Geometry: final body of the model. Coordinates: model frame, mm. A direction names the side the tool comes from. Round coordinates to 2 decimals unless told otherwise and drop trailing zeros. Order: outer loops, then holes, each group sorted by start corner. A loop starts at its lowest first (then second) coordinate and runs counter-clockwise, first axis right, second up. Notation, with made-up numbers: (34.25, -10.75) -> (61.25, -10.75) arc R23 ccw to (61.25, 9.25) -> close; hole circle Ø6 at (41.25, 7.25). An arc over 180 degrees is marked (long way). Put each result on its own line as item: value.
```python
from build123d import *

# Parameters (mm, degrees)
SHELL5_T         = 1
SWEEP1_PROFILE_R = 2.5


with BuildPart() as part:
    # Sketch1 → Revolve1 (revolve)
    with BuildSketch(Plane.XY, mode=Mode.PRIVATE) as revolve1_sk:
        Polygon((0, 620), (-126, 620), (-126, 610.763571771), (-131.422468228, 610.763571771), (-131.422468228, 606.763571771), (-126.257555316, 606.763571771), (-126.257555316, 591.763571771), (-131.422468228, 591.763571771), (-131.422468228, 587.763571771), (-126.257555316, 587.763571771), (-111.609923626, 0), (0, 0), align=None)
    revolve(revolve1_sk.sketch.rotate(Axis((0, 0, 0), (0, 1, 0)), 270), axis=Axis((0, 0, 0), (0, 1, 0)))

    # Shell5
    shell5_openings = [part.faces().sort_by_distance(p)[0] for p in [
        (0, 620, 0),
    ]]
    offset(amount=SHELL5_T, openings=shell5_openings, kind=Kind.INTERSECTION)

    # Sweep1: sweep along a path in Sketch4
    with BuildLine(Plane(origin=(0, 0, 0), x_dir=(1, 0, 0), z_dir=(0, 0, -1))) as sweep1_path:
        Line((-14.999820713, 0), (-14.999820713, -280.07351805))
        ThreePointArc((-14.999820713, -280.07351805), (0, -295.073338764), (14.999820713, -280.07351805))
        Line((14.999820713, -280.07351805), (14.999820713, -0.073338764))
    # Sweep1 profile (on start of the path) → Sweep1 (sweep)
    with BuildSketch(Plane(origin=(-14.999820713, 0, 0), x_dir=(1, 0, 0), z_dir=(0, 1, 0))):
        Circle(SWEEP1_PROFILE_R)
    sweep(path=sweep1_path.line)


solid = part.part
```
1. Cut plane B-B on y = 370.5. Return loops of the section in (x, z), and give its area (3 significant figures).
Ans:
outline: circle Ø243.69 at (0, 0); hole circle Ø241.69 at (0, 0)
area: 763 mm²
2. Cut plane C-C on y = 103. Return loops of the section in (x, z), and give its area (3 significant figures).
Ans:
outline: circle Ø230.35 at (0, 0); circle Ø5 at (-15, 0); circle Ø5 at (15, 0); hole circle Ø228.35 at (0, 0)
area: 760 mm²
3. Cut plane A-A on y = 263. Return loops of the section in (x, z), and give its area (3 significant figures).
Ans:
outline: circle Ø238.33 at (0, 0); circle Ø5 at (-15, 0); circle Ø5 at (15, 0); hole circle Ø236.33 at (0, 0)
area: 785 mm²
4. Contact query for flat-ended pins moving along their axis: P1, Ø2, axis at x = -25.5, y = 489.5, coming from the +Z side; P2, Ø2, axis at y = 170, z = -30.5, coming from the +X side; P3, Ø2, axis at y = 133.5, z = -28.5, coming from the -X side. Output: stop coordinate, or through.
Ans:
P1: z = 122.38
P2: x = 113.06
P3: x = -112.63
5. Draft query along Z for faces 5 (the face through (-126.175, 599.173, 16.566)), 6 (the face through (-2, -1, 2)), 7 (the face through (-117, 591.764, -49)). Return one class per face: +Z half, -Z half, draft (parallel to the pull), parting line (faces both ways), or undercut.
Ans:
face 5: parting line
face 6: draft
face 7: undercut
6. Set-up query: faces 1 (the face through (-131.3, 589.7, 17.2)), 2 (the face through (127, 611.764, 9)), 3 (the face through (116.96, 288.77, 25.97)), 4 (the face through (-69, 592.764, -109)). Return all of +Z, -Z, +X, -X, +Y, -Y with unobstructed straight access to the full face (end or side cutting, diameter ignored); none if empty.
Ans:
face 1: +Y, -Y
face 2: +Y
face 3: -Y
face 4: none
7. Material intervals for probe 1 along X at (y, z) = (614.75, 0); probe 2 along X at (y, z) = (608, 0); probe 3 along X at (y, z) = (97.5, -1), sorted ascending.
Ans:
probe 1: -127 to -126, 126 to 127
probe 2: -132.42 to -131.42, 131.42 to 132.42
probe 3: -115.04 to -114.04, -17.29 to -12.71, 12.71 to 17.29, 114.04 to 115.04
8. Cut plane D-D on y = 535.5. Return loops of the section in (x, z), and give its area (3 significant figures).
Ans:
outline: circle Ø251.91 at (0, 0); hole circle Ø249.91 at (0, 0)
area: 789 mm²
